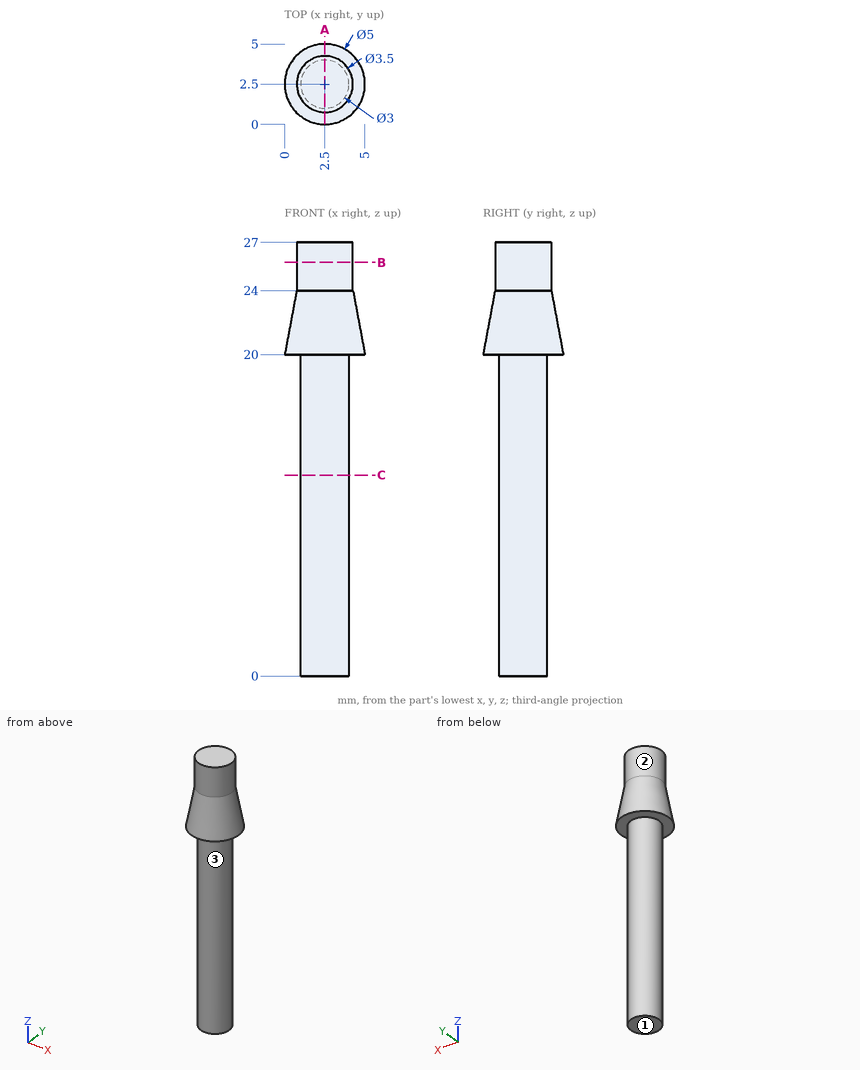
Input: dimensioned drawing with shaded views. Units: mm. Origin: part minimum x, y, z. A direction names the side the tool comes from. Coordinates: 2 decimals unless noted, no trailing zeros. Loops run counter-clockwise (first coordinate to the right, second up) from the corner with the lowest first, then second, coordinate; pieces in that order, holes last. Notation, with made-up numbers: M 75,25 L 114,25 A24 ccw 114,44 Z; hole C 70.5,35.25 d7. An arc over 180 degrees is marked long. Use a Markdown table: item, result. Add a question column.
Q1. Section query A-A, the plane x = 2.5. Return loops of the section in (y, z).
Q2. Section query C-C, the plane z = 12.5. Return loops of the section in (x, y).
Q3. First-contact query: pin 1 (1.5 mm diameter, centred on x = 1.5, y = 2, fed in from -Z); pin 2 (1 mm diameter, centred on x = 1.5, z = 3, fed in from +Y). Flat tips, straight axial feed; report the tip coordinate or a pass-through.
Q4. Material intervals for L1, parallel to Z at x = 2.2, y = 0.95; L2, parallel to Y at x = 2.55, z = 7.5; L3, parallel to Y at x = 3.8, z = 6.5, sorted ascending.
Q5. Access query for the marked faces 1, 2 and 3. Directions: +Z, -Z, +X, -X, +Y, -Y. A direction counts if a zero-diameter tool reaches every point of the face in a straight line with its end or side. Return the directions, or none.
Q6. Section query B-B, the plane z = 25.75. Return loops of the section in (x, y).
Result:
| question | item | result |
|---|---|---|
| 1 | outline | M 0,20 L 1,20 L 1,0 L 4,0 L 4,20 L 5,20 L 4.25,24 L 4.25,27 L 0.75,27 L 0.75,24 Z |
| 2 | outline | C 2.5,2.5 d3 |
| 3 | pin 1 | stops at z = 0 |
| 3 | pin 2 | stops at y = 3.91 |
| 4 | L1 | z = 20 to 27 |
| 4 | L2 | y = 1 to 4 |
| 4 | L3 | y = 1.75 to 3.25 |
| 5 | face 1 | -Z, +X, -X, +Y, -Y |
| 5 | face 2 | +Z |
| 5 | face 3 | -Z |
| 6 | outline | C 2.5,2.5 d3.5 |
